Input: part model. Units: mm. Frame: model coordinates. A direction names the side the tool comes from. Round coordinates to 2 decimals unless told otherwise and drop trailing zeros. Loops run counter-clockwise (first coordinate to the right, second up) from the corner with the lowest first, then second, coordinate; pieces in that order, holes last. Notation, with made-up numbers: (44, 19.25) -> (70, 19.25) arc R21 ccw to (70, 31.25) -> close; hole circle Ø6 at (29, -28). An arc over 180 degrees is marked (long way). Answer in a Markdown table with one row per item. Add a question column.
Q1. Section A-A, the plane x = -6.5. Output: boundary loops of the cut face in (y, z).
Q2. Mould query, pull axis Z, two halves, no side actions, for faces 1 (the face through (2.226, -14.066, 50.726)), 2 (the face through (11, -2, 35)), 3 (the face through (9, -9, 70)). Classes: pulls with the +Z half, pulls with the -Z half, needs draft (parallel to the pull), parting line crosses it, or undercut.
Q3. Section B-B, the plane z = 17.5. Output: boundary loops of the cut face in (x, y).
Q4. Reachability of faces 4 (the face through (7.81, -16.69, 20.5)), 5 (the face through (0.5, -16, 35)), 6 (the face through (-4, -17, 16)), 7 (the face through (-2.226, -13.914, 19.186)) from +Z, -Z, +X, -X, +Y, -Y: full face, straight path, thin tool, end or side. Return the list, or none.
Q5. Section D-D, the plane x = 10. Output: boundary loops of the cut face in (y, z), and give its area (3 significant figures).
Q6. Pin query (flat end, axial travel): pin 1 (1.5 mm diameter, centred on y = -3, z = 50.5, fed in from +X); pin 2 (7.5 mm diameter, centred on y = -13.5, z = 18, fed in from +X); pin 3 (3.5 mm diameter, centred on y = -16.5, z = 52, fed in from +X); pin 4 (10 mm diameter, centred on y = 1.5, z = 40, fed in from -X). Return the tip coordinate at first contact, or that it passes through.
Q7. Section C-C, the plane y = -1. Output: boundary loops of the cut face in (x, z).
Q8. Ray query, L1, parallel to Y at x = 2, z = 17; L2, parallel to X at y = 0, z = 16; L3, parallel to Z at x = -5.5, y = -16. Return the intervals inside material, ascending. Write a range as from..to.
```python
from build123d import *

# Parameters (mm, degrees)
SKETCH1_R                           = 20.5
SKETCH1_R_2                         = 11.5
BOSS_EXTRUDE1_DEPTH                 = 35
SKETCH2_R                           = 20.5
SKETCH2_R_2                         = 11
BOSS_EXTRUDE2_DEPTH                 = 35
CUT_EXTRUDE1_REACH                  = 77.766
SKETCH3_W                           = 1
SKETCH3_H                           = 20.5
CUT_EXTRUDE2_REACH                  = 77.766
CUT_EXTRUDE2_END_RADIUS             = 20.5
SKETCH4_R                           = 2
CUT_EXTRUDE2_DIRECTION_2_REACH      = 77.766
CUT_EXTRUDE2_DIRECTION_2_END_RADIUS = 20.5
CUT_EXTRUDE3_REACH                  = 78.945
CUT_EXTRUDE3_END_RADIUS             = 20.5
CUT_EXTRUDE4_REACH                  = 78.945
CUT_EXTRUDE4_END_RADIUS             = 20.5
SKETCH7_R                           = 3.6


with BuildPart() as part:
    # Sketch1 → Boss-Extrude1 (new body)
    with BuildSketch(Plane.XY):
        Circle(SKETCH1_R)
        Circle(SKETCH1_R_2, mode=Mode.SUBTRACT)
    extrude(amount=BOSS_EXTRUDE1_DEPTH)

    # Sketch2 → Boss-Extrude2 (add)
    with BuildSketch(Plane.XY.offset(35)):
        Circle(SKETCH2_R)
        Circle(SKETCH2_R_2, mode=Mode.SUBTRACT)
    extrude(amount=BOSS_EXTRUDE2_DEPTH)

    # Cut-Extrude1: up to this face of the body (flat: up to its plane)
    cut_extrude1_end = Plane(part.part.faces().sort_by_distance((-19.920172439, 0, 70))[0])
    # Sketch3 → Cut-Extrude1 (cut, up to the picked face)
    with BuildSketch(Plane(origin=(0, 0, 0), x_dir=(-1, 0, 0), z_dir=(0, 0, -1)), mode=Mode.PRIVATE) as cut_extrude1_sk1:
        with Locations((0, -10.25)):
            Rectangle(SKETCH3_W, SKETCH3_H)
    cut_extrude1_tool1 = split(extrude(cut_extrude1_sk1.sketch, amount=-CUT_EXTRUDE1_REACH, mode=Mode.PRIVATE), bisect_by=cut_extrude1_end, keep=Keep.BOTH, mode=Mode.PRIVATE)
    add(cut_extrude1_tool1.solids().sort_by(Axis((0, -10.25, 0), (0, 0, 1)))[0], mode=Mode.SUBTRACT)

    # Cut-Extrude2: up to this cylinder (the profile starts inside it)
    cut_extrude2_end = Plane(origin=(0, 0, 35), z_dir=(0, 0, -1)) * Cylinder(CUT_EXTRUDE2_END_RADIUS, 232.532, mode=Mode.PRIVATE)
    # Sketch4 → Cut-Extrude2 (cut, up to the surface)
    with BuildSketch(Plane(origin=(0, 0, 0), x_dir=(0, 0, -1), z_dir=(1, 0, 0)), mode=Mode.PRIVATE) as cut_extrude2_sk1:
        with Locations(Location((-52.5, -14.989125293, 0), (0, 0, 90))):
            Circle(SKETCH4_R)
    cut_extrude2_tool1 = extrude(cut_extrude2_sk1.sketch, amount=-CUT_EXTRUDE2_REACH, mode=Mode.PRIVATE) & cut_extrude2_end
    add(cut_extrude2_tool1.solids().sort_by_distance((0, -14.989125, 52.5))[0], mode=Mode.SUBTRACT)
    # Sketch4 → Cut-Extrude2 (cut, up to the surface)
    with BuildSketch(Plane(origin=(0, 0, 0), x_dir=(0, 0, -1), z_dir=(1, 0, 0)), mode=Mode.PRIVATE) as cut_extrude2_sk2:
        with Locations(Location((-17.5, -14.989125293, 0), (0, 0, 90))):
            Circle(SKETCH4_R)
    cut_extrude2_tool2 = extrude(cut_extrude2_sk2.sketch, amount=-CUT_EXTRUDE2_REACH, mode=Mode.PRIVATE) & cut_extrude2_end
    add(cut_extrude2_tool2.solids().sort_by_distance((0, -14.989125, 17.5))[0], mode=Mode.SUBTRACT)

    # Cut-Extrude2 direction 2: up to this cylinder (the profile starts inside it)
    cut_extrude2_direction_2_end = Plane(origin=(0, 0, 35), z_dir=(0, 0, -1)) * Cylinder(CUT_EXTRUDE2_DIRECTION_2_END_RADIUS, 232.532, mode=Mode.PRIVATE)
    # Sketch4 → Cut-Extrude2 direction 2 (cut, up to the surface)
    with BuildSketch(Plane(origin=(0, 0, 0), x_dir=(0, 0, -1), z_dir=(1, 0, 0)), mode=Mode.PRIVATE) as cut_extrude2_direction_2_sk1:
        with Locations(Location((-52.5, -14.989125293, 0), (0, 0, 90))):
            Circle(SKETCH4_R)
    cut_extrude2_direction_2_tool1 = extrude(cut_extrude2_direction_2_sk1.sketch, amount=CUT_EXTRUDE2_DIRECTION_2_REACH, mode=Mode.PRIVATE) & cut_extrude2_direction_2_end
    add(cut_extrude2_direction_2_tool1.solids().sort_by_distance((0, -14.989125, 52.5))[0], mode=Mode.SUBTRACT)
    # Sketch4 → Cut-Extrude2 direction 2 (cut, up to the surface)
    with BuildSketch(Plane(origin=(0, 0, 0), x_dir=(0, 0, -1), z_dir=(1, 0, 0)), mode=Mode.PRIVATE) as cut_extrude2_direction_2_sk2:
        with Locations(Location((-17.5, -14.989125293, 0), (0, 0, 90))):
            Circle(SKETCH4_R)
    cut_extrude2_direction_2_tool2 = extrude(cut_extrude2_direction_2_sk2.sketch, amount=CUT_EXTRUDE2_DIRECTION_2_REACH, mode=Mode.PRIVATE) & cut_extrude2_direction_2_end
    add(cut_extrude2_direction_2_tool2.solids().sort_by_distance((0, -14.989125, 17.5))[0], mode=Mode.SUBTRACT)

    # Cut-Extrude3: up to this cylinder (the profile starts inside it)
    cut_extrude3_end = Plane(origin=(0, 0, 35), z_dir=(0, 0, -1)) * Cylinder(CUT_EXTRUDE3_END_RADIUS, 234.89, mode=Mode.PRIVATE)
    # Sketch6 → Cut-Extrude3 (cut, up to the surface)
    with BuildSketch(Plane(origin=(4, 0, 0), x_dir=(0, 0, -1), z_dir=(1, 0, 0)), mode=Mode.PRIVATE) as cut_extrude3_sk1:
        Polygon((-48.516283143, -14.989125293), (-50.508141571, -11.539125293), (-54.491858429, -11.539125293), (-56.483716857, -14.989125293), (-54.491858429, -18.439125293), (-50.508141571, -18.439125293), align=None)
    cut_extrude3_tool1 = extrude(cut_extrude3_sk1.sketch, amount=CUT_EXTRUDE3_REACH, mode=Mode.PRIVATE) & cut_extrude3_end
    add(cut_extrude3_tool1.solids().sort_by_distance((4, -14.989125, 52.5))[0], mode=Mode.SUBTRACT)
    # Sketch6 → Cut-Extrude3 (cut, up to the surface)
    with BuildSketch(Plane(origin=(4, 0, 0), x_dir=(0, 0, -1), z_dir=(1, 0, 0)), mode=Mode.PRIVATE) as cut_extrude3_sk2:
        Polygon((-13.516283143, -14.989125293), (-15.508141571, -11.539125293), (-19.491858429, -11.539125293), (-21.483716857, -14.989125293), (-19.491858429, -18.439125293), (-15.508141571, -18.439125293), align=None)
    cut_extrude3_tool2 = extrude(cut_extrude3_sk2.sketch, amount=CUT_EXTRUDE3_REACH, mode=Mode.PRIVATE) & cut_extrude3_end
    add(cut_extrude3_tool2.solids().sort_by_distance((4, -14.989125, 17.5))[0], mode=Mode.SUBTRACT)

    # Cut-Extrude4: up to this cylinder (the profile starts inside it)
    cut_extrude4_end = Plane(origin=(0, 0, 35), z_dir=(0, 0, -1)) * Cylinder(CUT_EXTRUDE4_END_RADIUS, 234.89, mode=Mode.PRIVATE)
    # Sketch7 → Cut-Extrude4 (cut, up to the surface)
    with BuildSketch(Plane(origin=(-4, 0, 0), x_dir=(0, 0, -1), z_dir=(1, 0, 0)), mode=Mode.PRIVATE) as cut_extrude4_sk1:
        with Locations((-52.5, -14.989125293)):
            Circle(SKETCH7_R)
    cut_extrude4_tool1 = extrude(cut_extrude4_sk1.sketch, amount=-CUT_EXTRUDE4_REACH, mode=Mode.PRIVATE) & cut_extrude4_end
    add(cut_extrude4_tool1.solids().sort_by_distance((-4, -14.989125, 52.5))[0], mode=Mode.SUBTRACT)
    # Sketch7 → Cut-Extrude4 (cut, up to the surface)
    with BuildSketch(Plane(origin=(-4, 0, 0), x_dir=(0, 0, -1), z_dir=(1, 0, 0)), mode=Mode.PRIVATE) as cut_extrude4_sk2:
        with Locations((-17.5, -14.989125293)):
            Circle(SKETCH7_R)
    cut_extrude4_tool2 = extrude(cut_extrude4_sk2.sketch, amount=-CUT_EXTRUDE4_REACH, mode=Mode.PRIVATE) & cut_extrude4_end
    add(cut_extrude4_tool2.solids().sort_by_distance((-4, -14.989125, 17.5))[0], mode=Mode.SUBTRACT)


solid = part.part
```
Answer block:
| question | item | result |
|---|---|---|
| 1 | outline | (-19.44, 0) -> (-9.49, 0) -> (-9.49, 35) -> (-8.87, 35) -> (-8.87, 70) -> (-19.44, 70) -> close; (8.87, 35) -> (9.49, 35) -> (9.49, 0) -> (19.44, 0) -> (19.44, 70) -> (8.87, 70) -> close; hole circle Ø7.2 at (-14.99, 17.5); hole circle Ø7.2 at (-14.99, 52.5) |
| 2 | face 1 | undercut |
| 2 | face 2 | pulls with the -Z half |
| 2 | face 3 | pulls with the +Z half |
| 3 | outline | (-17.05, -11.39) -> (-4, -11.39) -> (-4, -12.99) -> (-0.5, -12.99) -> (-0.5, -11.49) arc R11.5 cw (long way) to (0.5, -11.49) -> (0.5, -12.99) -> (4, -12.99) -> (4, -11.54) -> (16.94, -11.54) arc R20.5 ccw (long way) to start; (-8.64, -18.59) arc R20.5 ccw to (-0.5, -20.49) -> (-0.5, -16.99) -> (-4, -16.99) -> (-4, -18.59) -> close; (0.5, -20.49) arc R20.5 ccw to (8.96, -18.44) -> (4, -18.44) -> (4, -16.99) -> (0.5, -16.99) -> close |
| 4 | face 4 | +X |
| 4 | face 5 | +Z, -Z, -Y |
| 4 | face 6 | -X |
| 4 | face 7 | +X, -X |
| 5 | outline | (-17.9, 0) -> (-5.68, 0) -> (-5.68, 35) -> (-4.58, 35) -> (-4.58, 70) -> (-17.9, 70) -> (-17.9, 54.81) -> (-14.99, 56.48) -> (-11.54, 54.49) -> (-11.54, 50.51) -> (-14.99, 48.52) -> (-17.9, 50.19) -> (-17.9, 19.81) -> (-14.99, 21.48) -> (-11.54, 19.49) -> (-11.54, 15.51) -> (-14.99, 13.52) -> (-17.9, 15.19) -> close; (4.58, 35) -> (5.68, 35) -> (5.68, 0) -> (17.9, 0) -> (17.9, 70) -> (4.58, 70) -> close |
| 5 | area | 1,710 mm^2 |
| 6 | pin 1 | x = 20.38 |
| 6 | pin 2 | x = 18.03 |
| 6 | pin 3 | x = 4 |
| 6 | pin 4 | x = -20.5 |
| 7 | outline | (-20.48, 0) -> (-11.46, 0) -> (-11.46, 35) -> (-10.95, 35) -> (-10.95, 70) -> (-20.48, 70) -> close; (10.95, 35) -> (11.46, 35) -> (11.46, 0) -> (20.48, 0) -> (20.48, 70) -> (10.95, 70) -> close |
| 8 | L1 | -20.4..-16.93, -13.05..-11.32, 11.32..20.4 |
| 8 | L2 | -20.5..-11.5, 11.5..20.5 |
| 8 | L3 | 0..14.04, 20.96..49.04, 55.96..70 |
